CAD build for the part. Positions are in the model's coordinates, mm. Face numbers are marked on the shaded views. A direction names the side the tool comes from. Give positions to 0.01 mm unless a question says otherwise; leave off trailing zeros. Loops run counter-clockwise (first coordinate to the right, second up) from the corner with the lowest first, then second, coordinate; pieces in that order, holes last. Notation, with made-up numbers: (57.25, -25.5) -> (115.25, -25.5) arc R9 ccw to (115.25, -18.5) -> close; hole circle Ø3 at (54.5, 68.25). An arc over 180 degrees is marked (long way). Write each question's results on one line, items separated by ' | '. Start each with the question number.
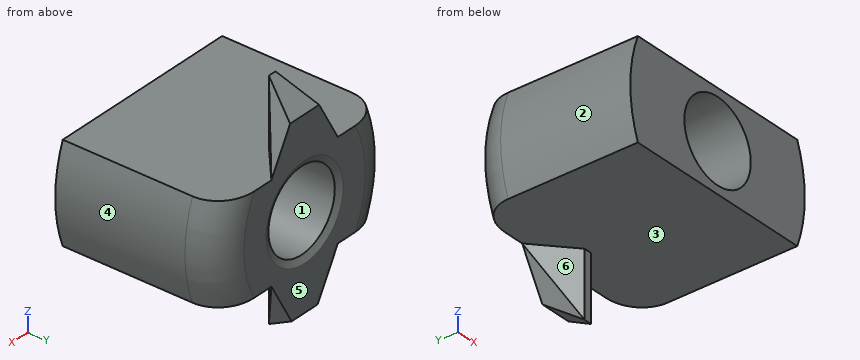
```python
from build123d import *

# Parameters (mm, degrees)
SALIENTE_EXTRUIR1_DEPTH   = 10
CROQUIS2_R                = 2.5
CORTAR_EXTRUIR1_DEPTH     = 10
CHAFL_N1_SIZE             = 0.4
CHAFL_N1_SIZE2            = 0.186523063
SALIENTE_EXTRUIR2_DEPTH   = 2
CORTAR_EXTRUIR2_START     = 0.687515582
CORTAR_EXTRUIR2_OUTLINE_W = 5
CORTAR_EXTRUIR2_OUTLINE_H = 5
CORTAR_EXTRUIR2_DEPTH     = 2.312484418
CORTAR_EXTRUIR4_DEPTH     = 9.799366623
CORTAR_EXTRUIR5_DEPTH     = 4
CORTAR_EXTRUIR6_START     = 19.504007809
CORTAR_EXTRUIR6_OUTLINE_W = 5
CORTAR_EXTRUIR6_OUTLINE_H = 5
CORTAR_EXTRUIR6_DEPTH     = 1.2
REDONDEO1_R               = 2


with BuildPart() as part:
    # Croquis1 → Saliente-Extruir1 (new body)
    with BuildSketch(Plane(origin=(0, 0, 0), x_dir=(1, 0, 0), z_dir=(0, 1, 0))):
        with BuildLine():
            Line((4.858013613, -14.380009761), (4.858013613, -8.380009761))
            Line((4.858013613, -8.380009761), (-1.141986387, -8.380009761))
            ThreePointArc((-1.141986387, -8.380009761), (-1.707193124, -11.380009761), (-1.141986387, -14.380009761))
            Line((-1.141986387, -14.380009761), (4.858013613, -14.380009761))
        make_face()
        with BuildLine():
            Line((10.858013613, -8.380009761), (4.858013613, -8.380009761))
            Line((4.858013613, -8.380009761), (4.858013613, -14.380009761))
            Line((4.858013613, -14.380009761), (10.858013613, -14.380009761))
            ThreePointArc((10.858013613, -14.380009761), (11.423220351, -11.380009761), (10.858013613, -8.380009761))
        make_face()
    extrude(amount=SALIENTE_EXTRUIR1_DEPTH)

    # Croquis2 → Cortar-Extruir1 (cut)
    with BuildSketch(Plane(origin=(0, 10, 0), x_dir=(1, 0, 0), z_dir=(0, 1, 0))):
        with Locations(Location((4.858013613, -11.380009761, 0), (0, 0, 270))):
            Circle(CROQUIS2_R)
    extrude(amount=-CORTAR_EXTRUIR1_DEPTH, mode=Mode.SUBTRACT)

    # Chaflán1
    chafl_n1_edges = [part.edges().sort_by_distance(p)[0] for p in [
        (4.858013613, 10, 8.880009761),
    ]]
    chafl_n1_side = [part.faces().sort_by_distance(p)[0] for p in [
        (4.858013613, 10, 8.524373107),
    ]]
    chamfer(chafl_n1_edges, length=CHAFL_N1_SIZE, length2=CHAFL_N1_SIZE2, reference=chafl_n1_side[0])

    # Croquis3 → Saliente-Extruir2 (add)
    with BuildSketch(Plane(origin=(0, 10, 0), x_dir=(1, 0, 0), z_dir=(0, 1, 0))):
        Polygon((2.358013613, -8.380009761), (4.858013613, -8.380009761), (4.858013613, -4.380009761), (4.608013613, -4.380009761), align=None)
        Polygon((4.858013613, -4.380009761), (4.858013613, -8.380009761), (7.358013613, -8.380009761), (5.108013613, -4.380009761), align=None)
    saliente_extruir2 = extrude(amount=-SALIENTE_EXTRUIR2_DEPTH)

    # Cortar-Extruir2: read off the stored shape, not the designer's step
    # Cortar-Extruir2 outline → Cortar-Extruir2 (cut)
    with BuildSketch(Plane(origin=(0, 0, 0), x_dir=(1, 0, 0), z_dir=(0, 0.5449883505954141, -0.8384436163006372)).offset(CORTAR_EXTRUIR2_START)):
        with Locations((4.5, -10.5)):
            Rectangle(CORTAR_EXTRUIR2_OUTLINE_W, CORTAR_EXTRUIR2_OUTLINE_H)
    extrude(amount=CORTAR_EXTRUIR2_DEPTH, mode=Mode.SUBTRACT)

    # Cortar-Extruir4: read off the stored shape, not the designer's step
    # Cortar-Extruir4 outline → Cortar-Extruir4 (cut)
    with BuildSketch(Plane(origin=(-1.717842267, 1.932572551, 0), x_dir=(-0.7474093186836599, -0.6643638388299198, 0), z_dir=(0.6643638388299198, -0.7474093186836599, 0))):
        Polygon((-9.132687685, -4.380009761), (-12.14308633, -8.380009761), (-9.132687685, -8.380009761), align=None)
    cortar_extruir4 = extrude(amount=CORTAR_EXTRUIR4_DEPTH, mode=Mode.SUBTRACT)

    # Croquis13 → Cortar-Extruir5 (cut, along a direction that is not the sketch's normal)
    with BuildSketch(Plane(origin=(6.006295664, 6.757082622, 0), x_dir=(0.7474093186836596, -0.66436383882992, 0), z_dir=(0.66436383882992, 0.7474093186836596, 0))):
        Polygon((-1.870838395, -8.380009761), (-1.870838395, -4.380009761), (-4.88123704, -8.380009761), align=None)
    cortar_extruir5 = extrude(amount=-CORTAR_EXTRUIR5_DEPTH, dir=(0, 1, 0), mode=Mode.SUBTRACT)

    # Simetría1: Saliente-Extruir2 across plane
    add(saliente_extruir2.mirror(Plane(origin=(0, 0, 11.380009761), x_dir=(1, 0, 0), z_dir=(0, 0, -1))))

    # Simetría3: Cortar-Extruir4, Cortar-Extruir5 across plane
    add(cortar_extruir4.mirror(Plane(origin=(0, 0, 11.380009761), x_dir=(1, 0, 0), z_dir=(0, 0, -1))), mode=Mode.SUBTRACT)
    add(cortar_extruir5.mirror(Plane(origin=(0, 0, 11.380009761), x_dir=(1, 0, 0), z_dir=(0, 0, -1))), mode=Mode.SUBTRACT)

    # Cortar-Extruir6: read off the stored shape, not the designer's step
    # Cortar-Extruir6 outline → Cortar-Extruir6 (cut)
    with BuildSketch(Plane(origin=(0, 0, 0), x_dir=(1, 0, 0), z_dir=(0, 0.5999999999999971, 0.8000000000000023)).offset(CORTAR_EXTRUIR6_START)):
        with Locations((4.5, -3.5)):
            Rectangle(CORTAR_EXTRUIR6_OUTLINE_W, CORTAR_EXTRUIR6_OUTLINE_H)
    extrude(amount=CORTAR_EXTRUIR6_DEPTH, mode=Mode.SUBTRACT)

    # Redondeo1
    redondeo1_edges = [part.edges().sort_by_distance(p)[0] for p in [
        (-1.707193124, 10, 11.380009761),
        (11.423220351, 10, 11.380009761),
    ]]
    fillet(redondeo1_edges, radius=REDONDEO1_R)


solid = part.part
```
Q1. Drop flat-ended pins along their axis: pin 1 (0.6 mm diameter, centred on x = 5, z = 15.5, fed in from -Y); pin 2 (1 mm diameter, centred on x = -0.5, y = 8.5, fed in from -Z); pin 3 (5 mm diameter, centred on y = 8, z = 16.5, fed in from -X); pin 4 (1 mm diameter, centred on y = 2, z = 15, fed in from -X). Give the stop position or say it passes through.
Q2. Saw through at B-B, the plane y = 2.5. List the corners of the cut face in (x, z), then the cut area to 3 significant figures.
Q3. Saw through at A-A, the plane z = 7.5. List the corners of the cut face in (x, y), then the cut area to 3 significant figures.
Q4. Wall check: L1, parallel to Z at x = 8.5, y = 7; L2, parallel to Z at x = 4.75, y = 0.75; L3, parallel to X at y = 2.75, z = 13. Give the ranges that are in metal, low to high.
Q5. Which spindle directions (+Z, -Z, +X, -X, +Y, -Y) get a long thin tool onto all of the face, cutting with end or side? Do the marked faces 5 and 6. Say none if no direction does.
Q6. Mould opens along X. For the marked faces 1, 2, 3 and 4 say: pulls with the +X half, pulls with the -X half, needs draft (parallel to the pull), parting line crosses it, or undercut.
Answer block:
1) pin 1: stops at y = 8 | pin 2: stops at z = 8.38 | pin 3: stops at x = -1.28 | pin 4: passes through
2) outline: (-1.14, 8.38) -> (10.86, 8.38) arc R8.24 ccw to (10.86, 14.38) -> (-1.14, 14.38) arc R8.24 ccw to start; hole circle Ø5 at (4.86, 11.38) | area: 56.9 mm2
3) outline: (2.85, 9.56) -> (4.61, 8) -> (5.11, 8) -> (6.86, 9.56) -> (6.86, 10) -> (2.85, 10) -> close | area: 5.28 mm2
4) L1: z = 8.38 to 14.38 | L2: z = 8.38 to 8.88, 13.88 to 14.38 | L3: x = -1.55 to 2.95, 6.76 to 11.26
5) face 5: +Z, -Z, +X, -X, +Y | face 6: -Z, -X, -Y
6) face 1: undercut | face 2: pulls with the -X half | face 3: needs draft | face 4: pulls with the +X half
